Could you check a few things on this model? Use its own coordinates, in mm. A direction names the side the tool comes from. Round coordinates to 2 decimals unless told otherwise and drop trailing zeros. Write each loop counter-clockwise with the first axis right and the second up, starting at its lowest first coordinate (ties: lowest second). Pieces come first, ordered by that corner, then holes. Notation, with made-up numbers: (55.25, 40) -> (102.25, 40) arc R26 cw to (102.25, 65) -> close; hole circle Ø5 at (-6.5, 44.25). An arc over 180 degrees is marked (long way). Answer as CSV lines item,"result". Start each with the question number.
Q1. Imagine slicing it at D-D on y = 2.95. Please give me the cut outline in (x, z), and give its area (3 significant figures).
Q2. If we mould it in two halves opening along X, with no side actions, what happens to faces 4 (the flat face through (-2, 1.9, -4)), 5 (the flat face through (0, 2, -2.4))? For each: pulls with the +X half, pulls with the -X half, needs draft (parallel to the pull), parting line crosses it, or undercut.
Q3. Imagine slicing it at A-A on x = 2. Please give me the cut outline in (y, z), and give its area (3 significant figures).
Q4. For faces 1 (the flat face through (2, 1.9, -4)), 2 (the cylindrical face through (0.02, 2.85, 0.2)), 3 (the cylindrical face through (1.199, 2.071, -2.685)), which set-ups out of +Z, -Z, +X, -X, +Y, -Y let a thin tool reach every point of the face, with its end or its side?
Q5. Will these pins go through, and if not, where does the flat tip stop? pin 1 Ø1.6 at (x, z) = (0.5, 1) entering from +Y; pin 2 Ø1.1 at (x, y) = (0, 1.5) entering from -Z; pin 3 Ø0.6 at (x, y) = (-5, 1) entering from +Z.
Q6. If I drill on line 1 (X direction, y = 3.15, z = 0.25); line 2 (Z direction, x = 1.75, y = 2); line 3 (X direction, y = 0.8, z = 0.5), over which ranges is the centre line in solid material (lowest first)? Write a range as [from, to].
Q7. Imagine slicing it at B-B on x = 0. Please give me the cut outline in (y, z), and give its area (3 significant figures).
Q8. Imagine slicing it at C-C on y = 2.2. Please give me the cut outline in (x, z), and give its area (3 significant figures).
from build123d import *

# Parameters (mm, degrees)
EXTRUDE_1_DEPTH     = 4.2
CHAMFER_1_SIZE      = 0.7
SKETCH_2_W          = 1.2
SKETCH_2_H          = 0.4
CUT_EXTRUDE_1_DEPTH = 7.4
SKETCH_3_W          = 0.2
SKETCH_3_H          = 0.5
EXTRUDE_2_DEPTH     = 0.4
SKETCH_4_W          = 0.2
SKETCH_4_H          = 0.5
SKETCH_5_W          = 0.2
SKETCH_5_H          = 0.5


with BuildPart() as part:
    # Эскиз1 → Бобышка-Вытянуть1 (new body)
    with BuildSketch(Plane(origin=(0, 0, 0), x_dir=(1, 0, 0), z_dir=(0, 1, 0))):
        with BuildLine():
            Line((-3.2, 0), (-3.2, 5.2))
            Line((-3.2, 5.2), (-1.5, 5.2))
            Line((-1.5, 5.2), (-1.5, 3.4))
            ThreePointArc((-1.5, 3.4), (-1.207106781, 2.692893219), (-0.5, 2.4))
            Line((-0.5, 2.4), (0.5, 2.4))
            ThreePointArc((0.5, 2.4), (1.207106781, 2.692893219), (1.5, 3.4))
            Line((1.5, 3.4), (1.5, 5.2))
            Line((1.5, 5.2), (3.2, 5.2))
            Line((3.2, 5.2), (3.2, 0))
            Line((3.2, 0), (-3.2, 0))
        make_face()
    extrude(amount=EXTRUDE_1_DEPTH)

    # Фаска1
    chamfer_1_edges = [part.edges().sort_by_distance(p)[0] for p in [
        (2.35, 4.2, -5.2),
        (-2.35, 4.2, -5.2),
    ]]
    chamfer(chamfer_1_edges, length=CHAMFER_1_SIZE)

    # Эскиз2 → Вырез-Вытянуть1 (cut, through all)
    with BuildSketch(Plane.ZY.offset(3.2)):
        with Locations((-4, 2.1)):
            Rectangle(SKETCH_2_W, SKETCH_2_H)
    extrude(amount=-CUT_EXTRUDE_1_DEPTH, mode=Mode.SUBTRACT)

    # Эскиз3 → Бобышка-Вытянуть2 (add)
    with BuildSketch(Plane.XY):
        with BuildLine():
            Line((-0.357071421, 3.7), (0.357071421, 3.7))
            ThreePointArc((0.357071421, 3.7), (0, 2.85), (-0.357071421, 3.7))
        make_face()
        with BuildLine():
            Line((-0.606217783, 0.5), (0.606217783, 0.5))
            ThreePointArc((0.606217783, 0.5), (0, 1.55), (-0.606217783, 0.5))
        make_face()
        with Locations((-2.5, 3.35)):
            Rectangle(SKETCH_3_W, SKETCH_3_H)
        with Locations((2.5, 3.35)):
            Rectangle(SKETCH_3_W, SKETCH_3_H)
        with Locations((2.5, 0.85)):
            Rectangle(SKETCH_3_W, SKETCH_3_H)
        with Locations((-2.5, 0.85)):
            Rectangle(SKETCH_3_W, SKETCH_3_H)
    extrude(amount=EXTRUDE_2_DEPTH)

    # По траектории1: sweep along a curve in space
    with BuildLine() as sweep_1_path:
        Line((2.4, 3.1, 0.4), (2.4, 3.1, 1.033279954))
        ThreePointArc((2.2, 3.1, 1.233279954), (2.341421356, 3.1, 1.17470131), (2.4, 3.1, 1.033279954))
        Line((2.2, 3.1, 1.233279954), (-3.1, 3.1, 1.233279954))
    # Эскиз4 → По траектории1 (sweep)
    with BuildSketch(Plane.XY.offset(0.4)):
        with Locations((2.5, 3.35)):
            Rectangle(SKETCH_4_W, SKETCH_4_H)
        with Locations((2.5, 0.85)):
            Rectangle(SKETCH_4_W, SKETCH_4_H)
    sweep(path=sweep_1_path.line)

    # По траектории2: sweep along a curve in space
    with BuildLine() as sweep_2_path:
        Line((-2.6, 0.6, 0.4), (-2.6, 0.6, 0.5))
        ThreePointArc((-2.8, 0.6, 0.7), (-2.658578644, 0.6, 0.641421356), (-2.6, 0.6, 0.5))
        Line((-2.8, 0.6, 0.7), (-5.7, 0.6, 0.7))
    # Эскиз5 → По траектории2 (sweep)
    with BuildSketch(Plane.XY.offset(0.4)):
        with Locations((-2.5, 3.35)):
            Rectangle(SKETCH_5_W, SKETCH_5_H)
        with Locations((-2.5, 0.85)):
            Rectangle(SKETCH_5_W, SKETCH_5_H)
    sweep(path=sweep_2_path.line)


solid = part.part
Checks:
1,outline,"(-3.2, -5.2) -> (-1.5, -5.2) -> (-1.5, -3.4) arc R1 cw to (-0.5, -2.4) -> (0.5, -2.4) arc R1 cw to (1.5, -3.4) -> (1.5, -5.2) -> (3.2, -5.2) -> (3.2, 0) -> (0.3, 0) -> (0.3, 0.4) -> (-0.3, 0.4) -> (-0.3, 0) -> (-3.2, 0) -> close"
1,area,"25.5 mm^2"
2,face 4,"needs draft"
2,face 5,"undercut"
3,outline,"(0, -5.2) -> (3.5, -5.2) -> (4.2, -4.5) -> (4.2, 0) -> (0, 0) -> close; (0.6, 1.23) -> (1.1, 1.23) -> (1.1, 1.43) -> (0.6, 1.43) -> close; (3.1, 1.23) -> (3.6, 1.23) -> (3.6, 1.43) -> (3.1, 1.43) -> close; hole (1.9, -4.6) -> (2.3, -4.6) -> (2.3, -3.4) -> (1.9, -3.4) -> close"
3,area,"21.3 mm^2"
4,face 1,"+X, -X"
4,face 2,"none"
4,face 3,"-Z, +Y, -Y"
5,pin 1,"y = 3.7"
5,pin 2,"z = -2.4"
5,pin 3,"z = 0.9"
6,line 1,"[-2.6, -2.4], [-0.46, 0.46], [2.4, 2.6]"
6,line 2,"[-5.2, -4.6], [-3.4, 0]"
6,line 3,"[-2.6, -2.4], [2.4, 2.6]"
7,outline,"(0, -2.4) -> (4.2, -2.4) -> (4.2, 0) -> (3.7, 0) -> (3.7, 0.4) -> (2.85, 0.4) -> (2.85, 0) -> (1.55, 0) -> (1.55, 0.4) -> (0.5, 0.4) -> (0.5, 0) -> (0, 0) -> close; (0.6, 1.23) -> (1.1, 1.23) -> (1.1, 1.43) -> (0.6, 1.43) -> close; (3.1, 1.23) -> (3.6, 1.23) -> (3.6, 1.43) -> (3.1, 1.43) -> close"
7,area,"11.0 mm^2"
8,outline,"(-3.2, -5.2) -> (-1.5, -5.2) -> (-1.5, -4.6) -> (-3.2, -4.6) -> close; (-3.2, -3.4) -> (-1.5, -3.4) arc R1 cw to (-0.5, -2.4) -> (0.5, -2.4) arc R1 cw to (1.5, -3.4) -> (3.2, -3.4) -> (3.2, 0) -> (-3.2, 0) -> close; (1.5, -5.2) -> (3.2, -5.2) -> (3.2, -4.6) -> (1.5, -4.6) -> close"
8,area,"21.2 mm^2"
